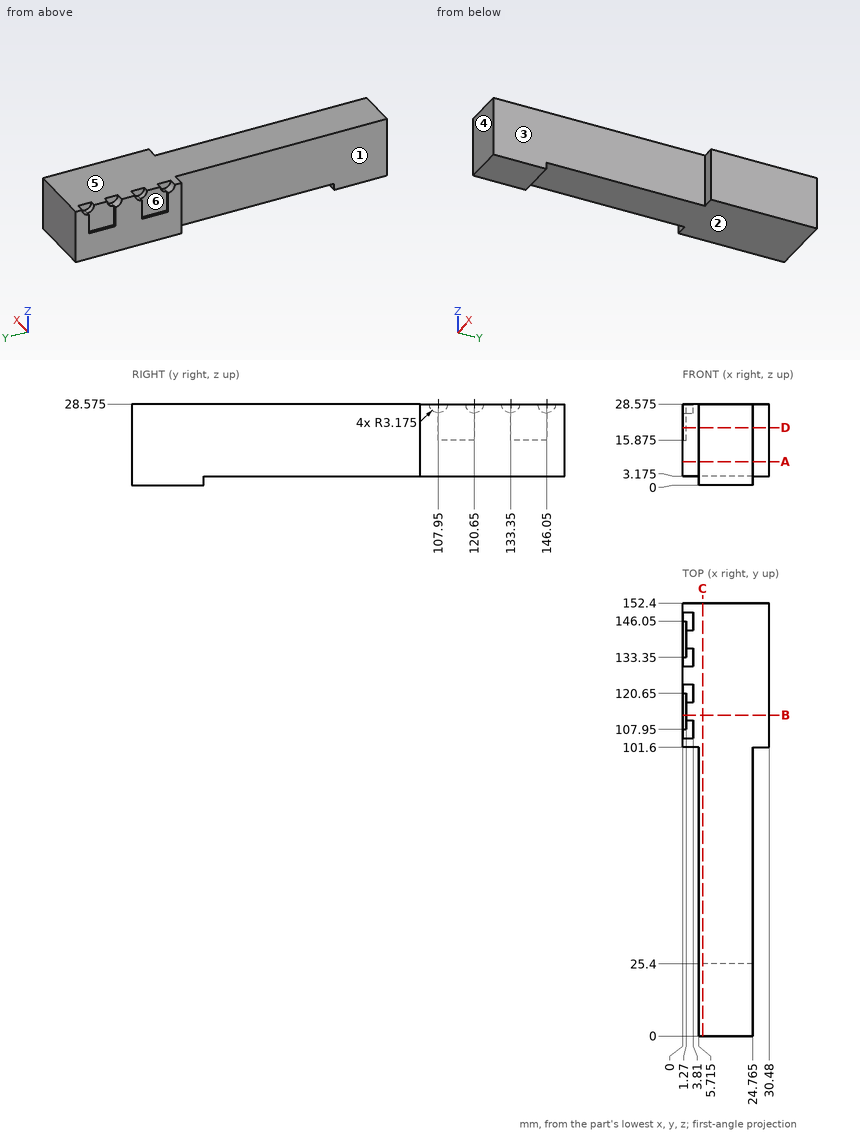
The drawing under review shows one solid part. Ordinate dimensions are in mm from its lowest x, y, z. A direction names the side the tool comes from. Round coordinates to 2 decimals unless told otherwise and drop trailing zeros. Write each loop counter-clockwise with the first axis right and the second up, starting at its lowest first coordinate (ties: lowest second). Pieces come first, ordered by that corner, then holes. Notation, with made-up numbers: (12.25, 76) -> (45.25, 76) arc R10 cw to (45.25, 94) -> close; hole circle Ø1 at (50.25, 45.25). An arc over 180 degrees is marked (long way). One line per question, with ' | ' between items. Start each with the question number.
(1) Add section A-A, the plane z = 8.25. Write out the cut boundary in (x, y) (3 decimals).
(2) Insertion check: P1, Ø3.5, axis at y = 120, z = 27.5, coming from the -X side; P2, Ø4.5, axis at x = 2, z = 11.5, coming from the -Y side; P3, Ø1, axis at x = 20.5, y = 50, coming from the -Z side (3 decimals). Each pin has a flat end and moves straight along its axis. Give the tip position at first contact, or say it passes through.
(3) Add section B-B, the plane y = 113. Write out the cut boundary in (x, z) (3 decimals), plus the area to 3 significant figures.
(4) For line 1 along Y through (x, z) = (21.5, 1); line 2 along X through (y, z) = (120.5, 19.5); line 3 along Y through (x, z) = (3.5, 11), list the stretches that pass through material, from the lowest coordinate up. Write a range as from..to.
(5) Add section C-C, the plane x = 7. Write out the cut boundary in (y, z) (3 decimals), plus the area to 3 significant figures.
(6) Tool access review of the marked faces 1, 2 and 3: name each direction out of +Z, -Z, +X, -X, +Y, -Y from which nothing blocks a thin tool from reaching the whole face with its end or side.
(7) Add section D-D, the plane z = 20.25. Write out the cut boundary in (x, y) (3 decimals), plus the area to 3 significant figures.
(8) Mouldability with a two-part tool opening along Y and no side actions: class the marked faces 4, 5 and 6 as released by +Y, released by -Y, zero draft, split by the parting line, or undercut.
Answer list:
1) outline: (0, 101.6) -> (5.715, 101.6) -> (5.715, 0) -> (24.765, 0) -> (24.765, 101.6) -> (30.48, 101.6) -> (30.48, 152.4) -> (0, 152.4) -> close
2) P1: x = 3.81 | P2: y = 101.6 | P3: z = 3.175
3) outline: (0, 3.175) -> (30.48, 3.175) -> (30.48, 28.575) -> (1.27, 28.575) -> (1.27, 15.875) -> (0, 15.875) -> close | area: 758 mm²
4) line 1: 0..25.4 | line 2: 1.27..30.48 | line 3: 101.6..152.4
5) outline: (0, 0) -> (25.4, 0) -> (25.4, 3.175) -> (152.4, 3.175) -> (152.4, 28.575) -> (0, 28.575) -> close | area: 3,950 mm²
6) face 1: +Z, -Z, -X, -Y | face 2: -Z, +X, -X, +Y | face 3: +Z, -Z, +X, -Y
7) outline: (0, 101.6) -> (5.715, 101.6) -> (5.715, 0) -> (24.765, 0) -> (24.765, 101.6) -> (30.48, 101.6) -> (30.48, 152.4) -> (0, 152.4) -> (0, 146.05) -> (1.27, 146.05) -> (1.27, 133.35) -> (0, 133.35) -> (0, 120.65) -> (1.27, 120.65) -> (1.27, 107.95) -> (0, 107.95) -> close | area: 3,450 mm²
8) face 4: released by -Y | face 5: zero draft | face 6: undercut
